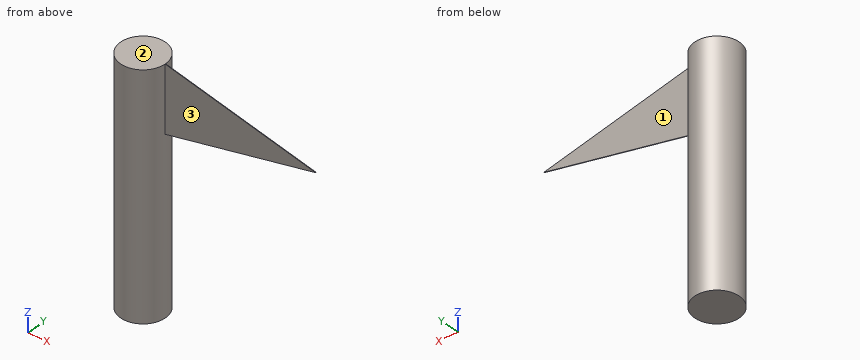
from build123d import *

# Parameters (mm, degrees)
F0_R     = 19.05
F1_DEPTH = 203.2
F3_DEPTH = 0.254


with BuildPart() as f1:
    # F0 (on Top) → F1 (new body)
    with BuildSketch(Plane.XY):
        Circle(F0_R)
    extrude(amount=F1_DEPTH)

    # F2 (on Front) → F3 (join, symmetric)
    with BuildSketch(Plane.XZ):
        Polygon((147.2438126802, 175.1202940941), (19.05, 203.2), (19.05, 147.0405881882), align=None)
        Polygon((19.05, 147.0405881882), (19.05, 203.2), (11.7504512891, 180.8726638556), align=None)
    extrude(amount=F3_DEPTH, both=True)


solid = f1.part
The listing builds one solid part. Answer for the finished solid, in the listing's coordinates (mm). Face numbers are marked on the shaded views. A direction names the side the tool comes from. Give positions to 0.01 mm unless a question says otherwise; leave off trailing zeros. Write each loop counter-clockwise with the first axis right and the second up, starting at its lowest first coordinate (ties: lowest second). Pieces come first, ordered by that corner, then holes.
1) Find the intervals of material crossed by L1, parallel to X at y = 14, z = 94; L2, parallel to X at y = -3, z = 190.5; L3, parallel to Y at x = 77, z = 168.5, in increasing order.
2) A tool of negligible diameter and unlimited length cuts with its end or side. For the marked faces 1, 2 and 3, from which of +Z, -Z, +X, -X, +Y, -Y can it reach the whole face along a straight path? Write none if from no direction.
3) Section C-C (y = -14) is taken. Write down the section's boundary in (x, z), and give its area (3 significant figures).
4) Given P1, Ø17, axis at x = 100, z = 180.5, coming from the +Y side; P2, Ø6, axis at y = -14, z = 147.5, coming from the +X side; P3, Ø12, axis at x = 19, y = -3, coming from the -Z side; P4, Ø6, axis at x = 20, z = 84, coming from the -Y side, each flat-ended and moving along its own axis, determine where each tip first touches the part or whether it passes through.
5) Section A-A (z = 90) is taken. Write down the section's boundary in (x, y), and give its area (3 significant figures).
6) Section B-B (x = 54.5) is taken. Write down the section's boundary in (y, z) (3 decimals).
Response:
1. L1: x = -12.92 to 12.92
1. L2: x = -18.81 to 18.81
1. L3: y = -0.25 to 0.25
2. face 1: +Z, -Z, +X, +Y
2. face 2: +Z, +X, -X, +Y, -Y
2. face 3: +Z, -Z, +X, -Y
3. outline: (-12.92, 0) - (12.92, 0) - (12.92, 203.2) - (-12.92, 203.2) - close
3. area: 5,250 mm2
4. P1: stops at y = 0.25
4. P2: stops at x = 15.55
4. P3: stops at z = 0
4. P4: stops at y = -8.6
5. outline: circle Ø38.1 at (0, 0)
5. area: 1,140 mm2
6. outline: (-0.254, 154.806) - (0.254, 154.806) - (0.254, 195.435) - (-0.254, 195.435) - close
